Geometry check sheet. Reference: the model listing, model coordinates, mm. A direction names the side the tool comes from. Coordinates: 2 decimals unless noted, no trailing zeros. Write each loop counter-clockwise with the first axis right and the second up, starting at its lowest first coordinate (ties: lowest second). Pieces come first, ordered by that corner, then holes. Notation, with made-up numbers: (14.5, 8.25) -> (73.5, 8.25) arc R16 ccw to (73.5, 20.25) -> close; hole circle Ø1 at (67.25, 26). An arc over 180 degrees is marked (long way). Answer in a Markdown table with one row per item. Add a question column.
Q1. Release check for a two-part mould opening along Z. For faces 1 (the face through (-26.344, -13, 35)), 2 (the face through (-48.326, -12.522, 9.851)), 3 (the face through (-64.604, -13, 42)) record: pulls with the +Z half, pulls with the -Z half, needs draft (parallel to the pull), parting line crosses it, or undercut.
Q2. Thickness scan on line 1 (Z direction, x = 0.5, y = -15.5); line 2 (Z direction, x = -46.5, y = -9); line 3 (Z direction, x = 82.5, y = -19.25). Record the ranges inside material, lowest first.
Q3. Tool access check on faces 4 (the face through (-53.916, -13, 35)), 5 (the face through (23, 0, 9)). Record the directions out of +Z, -Z, +X, -X, +Y, -Y that give a thin tool (end or side, any length) a straight path to the whole face; none if there is none.
Q4. Gauge pin test, flat ends, axial feed: P1, Ø5, axis at y = -3, z = -6, coming from the -X side; P2, Ø3, axis at y = -11, z = -8.5, coming from the +X side; P3, Ø1, axis at y = -12.5, z = 21.5, coming from the -X side. Record the tip position at first contact, or that the pin passes through.
Q5. Section check A-A, the plane y = -22.25. Count the separate pieces of the cut face and the enclosed holes in it, and give its area (3 significant figures).
Q6. Section check B-B, the plane x = 91.5. Record the boundary of the cut face in (y, z), and give its area (3 significant figures).
Q7. Section check C-C, the plane z = 14.5. Record the boundary of the cut face in (x, y).
Q8. Section check D-D, the plane x = 46.5. Record the boundary of the cut face in (y, z).
```python
from build123d import *

# Parameters (mm, degrees)
F0_R     = 17.986048
F0_R_2   = 8.517219
F1_DEPTH = 25.4


with BuildPart() as f1:
    # F0 (on Front) → F1 (new body)
    with BuildSketch(Plane.XZ):
        with BuildLine():
            Line((6.968918, 34.091828), (2.523895, 34.705166))
            ThreePointArc((2.523895, 34.705166), (1.262779, 34.773898), (0, 34.796818))
            ThreePointArc((0, 34.796818), (-29.316392, 18.744805), (-31.585075, -14.601425))
            ThreePointArc((-31.585075, -14.601425), (-13.574429, -32.039873), (11.482109, -32.847827))
            ThreePointArc((11.482109, -32.847827), (28.375689, -20.140478), (34.796818, 0))
            ThreePointArc((34.796818, 0), (26.956583, 22.003663), (6.968918, 34.091828))
        make_face()
        Circle(F0_R, mode=Mode.SUBTRACT)
        with BuildLine():
            ThreePointArc((6.968918, 34.091828), (4.756303, 34.470221), (2.523895, 34.705166))
            Line((2.523895, 34.705166), (6.968918, 34.091828))
        make_face()
        Polygon((-26.343811, 34.796818), (0, 34.796818), (-26.504347, 50.855222), (-26.504347, 41.345175), (-26.343811, 41.345175), align=None)
        with BuildLine():
            ThreePointArc((-31.585075, -14.601425), (-29.316392, 18.744805), (0, 34.796818))
            Line((0, 34.796818), (-26.343811, 34.796818))
            Line((-26.343811, 34.796818), (-26.343811, 27.887493))
            Line((-26.343811, 27.887493), (-53.915653, 27.887493))
            Line((-53.915653, 27.887493), (-53.915653, 33.627392))
            Line((-53.915653, 33.627392), (-64.604347, 33.627392))
            Line((-64.604347, 33.627392), (-31.585075, -14.601425))
        make_face()
        with BuildLine():
            Line((94.482827, 22.0164), (6.968918, 34.091828))
            ThreePointArc((6.968918, 34.091828), (26.956583, 22.003663), (34.796818, 0))
            ThreePointArc((34.796818, 0), (28.375689, -20.140478), (11.482109, -32.847827))
            Line((11.482109, -32.847827), (87.876434, -21.936645))
            ThreePointArc((87.876434, -21.936645), (69.466815, 3.303437), (94.482827, 22.0164))
        make_face()
        Polygon((-26.504347, 41.345175), (-26.504347, 50.855222), (-64.604347, 50.855222), (-64.604347, 33.627392), (-53.915653, 33.627392), (-53.915653, 41.345175), align=None)
        with BuildLine():
            ThreePointArc((113.669939, 0), (108.200053, 14.601944), (94.482827, 22.0164))
            ThreePointArc((94.482827, 22.0164), (69.466815, 3.303437), (87.876434, -21.936645))
            ThreePointArc((87.876434, -21.936645), (105.843561, -16.93016), (113.669939, 0))
        make_face()
        with Locations((91.444939, 0)):
            Circle(F0_R_2, mode=Mode.SUBTRACT)
    extrude(amount=F1_DEPTH)


solid = f1.part
```
Calculated:
| question | item | result |
|---|---|---|
| 1 | face 1 | undercut |
| 1 | face 2 | pulls with the -Z half |
| 1 | face 3 | needs draft |
| 2 | line 1 | z = -34.79 to -17.98, 17.98 to 34.79 |
| 2 | line 2 | z = 7.18 to 27.89, 41.35 to 50.86 |
| 2 | line 3 | z = -22.7 to 23.67 |
| 3 | face 4 | +Y, -Y |
| 3 | face 5 | +Z, -Z, +X, -X, +Y |
| 4 | P1 | stops at x = -39.19 |
| 4 | P2 | stops at x = 112.54 |
| 4 | P3 | stops at x = -56.64 |
| 5 | separate pieces | 1 |
| 5 | enclosed holes | 3 |
| 5 | area | 8,030 mm² |
| 6 | outline | (-25.4, -22.22) -> (0, -22.22) -> (0, -8.52) -> (-25.4, -8.52) -> close; (-25.4, 8.52) -> (0, 8.52) -> (0, 22.43) -> (-25.4, 22.43) -> close |
| 6 | area | 702 mm² |
| 7 | outline | (-51.51, -25.4) -> (-10.64, -25.4) -> (-10.64, 0) -> (-51.51, 0) -> close; (10.64, -25.4) -> (108.29, -25.4) -> (108.29, 0) -> (10.64, 0) -> close |
| 8 | outline | (-25.4, -27.85) -> (0, -27.85) -> (0, 28.64) -> (-25.4, 28.64) -> close |
